from build123d import *

# Parameters (mm, degrees)
SKETCH1_W           = 38.1
SKETCH1_H           = 38.1
SKETCH1_R           = 1.2
BOSS_EXTRUDE1_DEPTH = 1.6
BOSS_EXTRUDE2_DEPTH = 6.7
BOSS_EXTRUDE3_DEPTH = 5.7


with BuildPart() as part:
    # Sketch1 → Boss-Extrude1 (new body)
    with BuildSketch(Plane(origin=(0, 0, 0), x_dir=(1, 0, 0), z_dir=(0, 1, 0))):
        Rectangle(SKETCH1_W, SKETCH1_H)
        with Locations(Location((-17, 17, 0), (0, 0, 270))):
            Circle(SKETCH1_R, mode=Mode.SUBTRACT)
        with Locations(Location((17, 17, 0), (0, 0, 270))):
            Circle(SKETCH1_R, mode=Mode.SUBTRACT)
        with Locations(Location((17, -17, 0), (0, 0, 270))):
            Circle(SKETCH1_R, mode=Mode.SUBTRACT)
        with Locations(Location((-17, -17, 0), (0, 0, 270))):
            Circle(SKETCH1_R, mode=Mode.SUBTRACT)
    extrude(amount=BOSS_EXTRUDE1_DEPTH)

    # Sketch2 → Boss-Extrude2 (add)
    with BuildSketch(Plane(origin=(0, 1.6, 0), x_dir=(1, 0, 0), z_dir=(0, 1, 0))):
        with BuildLine():
            Line((-5, 13), (5, 13))
            ThreePointArc((5, 13), (9.949747468, 10.949747468), (12, 6))
            Line((12, 6), (12, -6))
            ThreePointArc((12, -6), (9.949747468, -10.949747468), (5, -13))
            Line((5, -13), (-5, -13))
            ThreePointArc((-5, -13), (-9.949747468, -10.949747468), (-12, -6))
            Line((-12, -6), (-12, 6))
            ThreePointArc((-12, 6), (-9.949747468, 10.949747468), (-5, 13))
        make_face()
    extrude(amount=BOSS_EXTRUDE2_DEPTH)

    # Sketch3 → Boss-Extrude3 (add)
    with BuildSketch(Plane(origin=(0, 8.3, 0), x_dir=(1, 0, 0), z_dir=(0, 1, 0))):
        with BuildLine():
            Line((7.030824987, 1.3), (7.95, 1.3))
            Line((7.95, 1.3), (7.95, -1.3))
            Line((7.95, -1.3), (7.030824987, -1.3))
            ThreePointArc((7.030824987, -1.3), (-7.15, 0), (7.030824987, 1.3))
        make_face()
    extrude(amount=BOSS_EXTRUDE3_DEPTH)


solid = part.part
The listing builds one solid part. Answer for the finished solid, in the listing's coordinates (mm). A direction names the side the tool comes from. Coordinates: 2 decimals unless noted, no trailing zeros. Order: outer loops, then holes, each group sorted by start corner. A loop starts at its lowest first (then second) coordinate and runs counter-clockwise, first axis right, second up.
Q1. A cutting plane is placed at D-D, the plane z = 0. Write down the section's boundary in (x, y), and give its area (3 significant figures).
Q2. A cutting plane is placed at C-C, the plane y = 4. Write down the section's boundary in (x, z).
Q3. A cutting plane is placed at B-B, the plane x = -17. Write down the section's boundary in (y, z), and give its area (3 significant figures).
Q4. Which of the six approach directions +Z, -Z, +X, -X, +Y, -Y give full straight-line access (tool end or side, diameter ignored) to faces 4 (the face through (-12, 5, 0)), 5 (the face through (-10, 4.9, -10.9)), 6 (the face through (7.5, 11.1, 1.3)), 7 (the face through (7.5, 11.1, -1.3))?
Q5. Consider line 1 (X direction, y = 0.45, z = 17); line 2 (Y direction, x = -13.5, z = 9.5); line 3 (Y direction, x = -8.5, z = -4). Determine where each line is inside the solid, lowest interval first.
Q6. For a pull along Z with two mould halves and no side action, classify faces 1 (the face through (-5, 8.3, -6)), 2 (the face through (15.83, 0.79, 16.74)), 3 (the face through (0, 5, -13)) as pulls with the +Z half, pulls with the -Z half, needs draft (parallel to the pull), parting line crosses it, or undercut.
Q7. A cutting plane is placed at A-A, the plane z = -17. Write down the section's boundary in (x, y), and give its area (3 significant figures).
Q8. Given P1, Ø3, axis at x = -17, z = -17, coming from the +Y side; P2, Ø5.5, axis at x = 0, y = 5, coming from the -Z side; P3, Ø0.7, axis at x = 7.5, y = 12.5, coming from the -Z side; P4, Ø1.5, axis at y = 10.5, z = -9.5, coming from the -X side, each flat-ended and moving along its own axis, determine where each tip first touches the part or whether it passes through.
Answers follow:
1. outline: (-19.05, 0) - (19.05, 0) - (19.05, 1.6) - (12, 1.6) - (12, 8.3) - (7.95, 8.3) - (7.95, 14) - (-7.15, 14) - (-7.15, 8.3) - (-12, 8.3) - (-12, 1.6) - (-19.05, 1.6) - close
1. area: 308 mm2
2. outline: (-12, -6) arc R7 ccw to (-5, -13) - (5, -13) arc R7 ccw to (12, -6) - (12, 6) arc R7 ccw to (5, 13) - (-5, 13) arc R7 ccw to (-12, 6) - close
3. outline: (0, -19.05) - (1.6, -19.05) - (1.6, -18.2) - (0, -18.2) - close; (0, -15.8) - (1.6, -15.8) - (1.6, 15.8) - (0, 15.8) - close; (0, 18.2) - (1.6, 18.2) - (1.6, 19.05) - (0, 19.05) - close
3. area: 53.3 mm2
4. face 4: +Z, -Z, -X, +Y
4. face 5: -Z, -X, +Y
4. face 6: +Z, +X, +Y
4. face 7: -Z, +X, +Y
5. line 1: x = -19.05 to -18.2, -15.8 to 15.8, 18.2 to 19.05
5. line 2: y = 0 to 1.6
5. line 3: y = 0 to 8.3
6. face 1: needs draft
6. face 2: undercut
6. face 3: pulls with the -Z half
7. outline: (-19.05, 0) - (-18.2, 0) - (-18.2, 1.6) - (-19.05, 1.6) - close; (-15.8, 0) - (15.8, 0) - (15.8, 1.6) - (-15.8, 1.6) - close; (18.2, 0) - (19.05, 0) - (19.05, 1.6) - (18.2, 1.6) - close
7. area: 53.3 mm2
8. P1: stops at y = 1.6
8. P2: stops at z = -13
8. P3: stops at z = -1.3
8. P4: passes through
